Study the drawing (mm; zero at the part's minimum x, y, z) and answer. A direction names the side the tool comes from. Coordinates: 2 decimals unless noted, no trailing zeros. Loops run counter-clockwise (first coordinate to the right, second up) from the corner with the lowest first, then second, coordinate; pieces in that order, holes last. Notation, with made-up numbers: (31, 30.5) -> (64, 30.5) arc R32 ccw to (64, 59.5) -> close; hole circle Ø7 at (38, 85.5). An arc over 180 degrees is marked (long way). One line per question, with ' | ' between items. Start each with the question number.
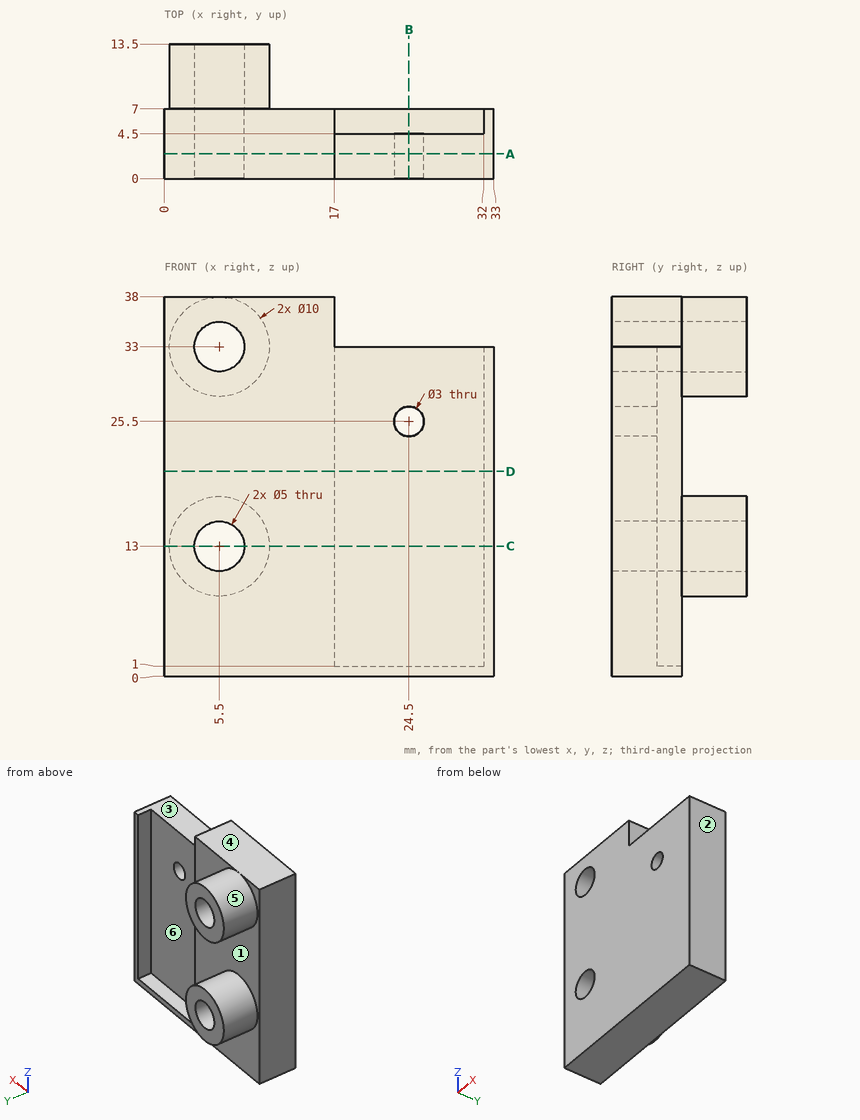
(1) Each of these flat-tipped pins is pushed along its axis until it touches: pin 1 Ø7.5 at (x, z) = (22.5, 10.5) entering from +Y; pin 2 Ø7.5 at (x, y) = (26.5, 2) entering from +Z; pin 3 Ø0.8 at (x, y) = (24, 5.5) entering from +Z. Where does it stop, or does it pass through?
(2) Determine the mould class of the marked faces 1, 2 and 3 for opening direction Z: +Z half, -Z half, draft (parallel to the pull), parting line (faces both ways), or undercut.
(3) Section C-C on z = 13 is taken. Write down the section's boundary in (x, y), plus the area to 3 significant figures.
(4) Find the intervals of material crossed by probe 1 along X at (y, z) = (1.5, 13); probe 2 along Z at (x, y) = (24.5, 3.2); probe 3 along X at (y, z) = (1, 25.5), in increasing order. Write a range as from..to.
(5) A tool of negligible diameter and unlimited length cuts with its end or side. For the marked faces 4, 5 and 6, from which of +Z, -Z, +X, -X, +Y, -Y can it reach the whole face along a straight path? Write none if from no direction.
(6) Section B-B on x = 24.5 is taken. Write down the section's boundary in (y, z), plus the area to 4 significant figures.
(7) Section A-A on y = 2.5 is taken. Write down the section's boundary in (x, z), plus the area to 3 significant figures.
(8) Section D-D on z = 20.5 is taken. Write down the section's boundary in (x, y), plus the area to 4 significant figures.
Working result:
1) pin 1: stops at y = 4.5 | pin 2: stops at z = 33 | pin 3: stops at z = 1
2) face 1: undercut | face 2: draft | face 3: +Z half
3) outline: (0, 0) -> (3, 0) -> (3, 13.5) -> (0.5, 13.5) -> (0.5, 7) -> (0, 7) -> close; (8, 0) -> (33, 0) -> (33, 7) -> (32, 7) -> (32, 4.5) -> (17, 4.5) -> (17, 7) -> (10.5, 7) -> (10.5, 13.5) -> (8, 13.5) -> close | area: 191 mm2
4) probe 1: x = 0..3, 8..33 | probe 2: z = 0..24, 27..33 | probe 3: x = 0..23, 26..33
5) face 4: +Z, +X, -X, +Y, -Y | face 5: +Y | face 6: +Z, +Y
6) outline: (0, 0) -> (7, 0) -> (7, 1) -> (4.5, 1) -> (4.5, 24) -> (0, 24) -> close; (0, 27) -> (4.5, 27) -> (4.5, 33) -> (0, 33) -> close | area: 137.5 mm2
7) outline: (0, 0) -> (33, 0) -> (33, 33) -> (17, 33) -> (17, 38) -> (0, 38) -> close; hole circle Ø5 at (5.5, 13); hole circle Ø5 at (5.5, 33); hole circle Ø3 at (24.5, 25.5) | area: 1,130 mm2
8) outline: (0, 0) -> (33, 0) -> (33, 7) -> (32, 7) -> (32, 4.5) -> (17, 4.5) -> (17, 7) -> (0, 7) -> close | area: 193.5 mm2
